from build123d import *

# Parameters (mm, degrees)
SKETCH1_R           = 14.2875
SKETCH1_R_2         = 2.4892
BOSS_EXTRUDE1_DEPTH = 2.54
FILLET1_R           = 7.62


with BuildPart() as part:
    # Sketch1 → Boss-Extrude1 (new body)
    with BuildSketch(Plane.XY):
        with BuildLine():
            Line((-76.2, -15.1892), (-76.2, -25.4))
            Line((-76.2, -25.4), (76.2, -25.4))
            Line((76.2, -25.4), (76.2, -15.1892))
            ThreePointArc((76.2, -15.1892), (73.7108, -12.7), (76.2, -10.2108))
            Line((76.2, -10.2108), (76.2, 133.35))
            Line((76.2, 133.35), (-76.2, 133.35))
            Line((-76.2, 133.35), (-76.2, -10.2108))
            ThreePointArc((-76.2, -10.2108), (-73.7108, -12.7), (-76.2, -15.1892))
        make_face()
        with Locations((0, 53.975)):
            Circle(SKETCH1_R, mode=Mode.SUBTRACT)
        with Locations((-63.5, -12.7)):
            Circle(SKETCH1_R_2, mode=Mode.SUBTRACT)
        with Locations((-50.8, -12.7)):
            Circle(SKETCH1_R_2, mode=Mode.SUBTRACT)
        with Locations((-38.1, -12.7)):
            Circle(SKETCH1_R_2, mode=Mode.SUBTRACT)
        with Locations((-25.4, -12.7)):
            Circle(SKETCH1_R_2, mode=Mode.SUBTRACT)
        with Locations((-12.7, -12.7)):
            Circle(SKETCH1_R_2, mode=Mode.SUBTRACT)
        with Locations((0, -12.7)):
            Circle(SKETCH1_R_2, mode=Mode.SUBTRACT)
        with Locations((12.7, -12.7)):
            Circle(SKETCH1_R_2, mode=Mode.SUBTRACT)
        with Locations((25.4, -12.7)):
            Circle(SKETCH1_R_2, mode=Mode.SUBTRACT)
        with Locations((38.1, -12.7)):
            Circle(SKETCH1_R_2, mode=Mode.SUBTRACT)
        with Locations((50.8, -12.7)):
            Circle(SKETCH1_R_2, mode=Mode.SUBTRACT)
        with Locations((63.5, -12.7)):
            Circle(SKETCH1_R_2, mode=Mode.SUBTRACT)
        with Locations((0, 109.855)):
            Circle(SKETCH1_R, mode=Mode.SUBTRACT)
    extrude(amount=BOSS_EXTRUDE1_DEPTH)

    # Fillet1
    fillet1_edges = [part.edges().sort_by_distance(p)[0] for p in [
        (76.2, -25.4, 1.27),
        (-76.2, -25.4, 1.27),
        (-76.2, 133.35, 1.27),
        (76.2, 133.35, 1.27),
    ]]
    fillet(fillet1_edges, radius=FILLET1_R)


solid = part.part
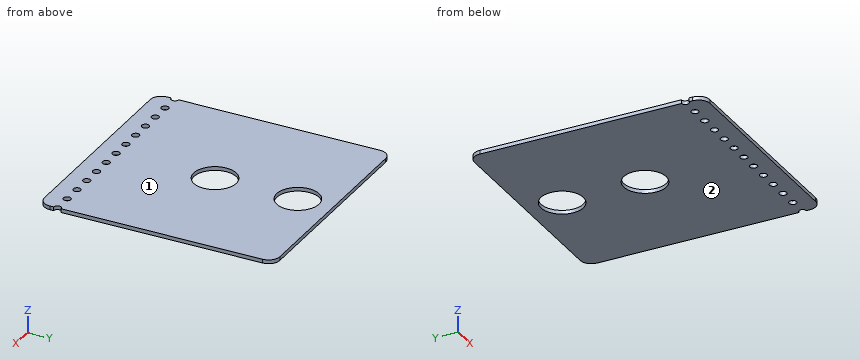
Design review of the part built by this model. Coordinates are the model's own, in mm. Face numbers are marked on the shaded views. Round coordinates to 2 decimals unless told otherwise and drop trailing zeros. Write each loop counter-clockwise with the first axis right and the second up, starting at its lowest first coordinate (ties: lowest second). Pieces come first, ordered by that corner, then holes. Notation, with made-up numbers: (-16.5, 23) - (-1.5, 23) arc R21 ccw to (-1.5, 58) - close; hole circle Ø10 at (71.5, 61.5). An arc over 180 degrees is marked (long way). Use a Markdown table: item, result. Add a question column.
1. We need section D-D (z = 1.1). Count the separate pieces of the cut face and the enclosed holes in it, then the cut area to 3 significant figures.
2. We need section A-A (x = -63.5). State the section outline as (y, z) points, then the cut area to 3 significant figures.
3. Wall thickness on probe 1 along Y at (x, z) = (0, 1.45); probe 2 along Y at (x, z) = (1, 1.4); probe 3 along Y at (x, z) = (-50.8, 1): over which ranges is each line inside the solid? List them lowest first.
4. We need section B-B (y = 46). State the section outline as (x, z) points.
5. Mouldability with a two-part tool opening along Z and no side actions: class the marked faces 1 and 2 as +Z half, -Z half, draft (parallel to the pull), parting line (faces both ways), or undercut.
6. We need section C-C (x = 0). State the section outline as (y, z) points, then the cut area to 3 significant figures.
Output:
| question | item | result |
|---|---|---|
| 1 | separate pieces | 1 |
| 1 | enclosed holes | 13 |
| 1 | area | 22,600 mm2 |
| 2 | outline | (-25.4, 0) - (-15.19, 0) - (-15.19, 2.54) - (-25.4, 2.54) - close; (-10.21, 0) - (133.35, 0) - (133.35, 2.54) - (-10.21, 2.54) - close |
| 2 | area | 391 mm2 |
| 3 | probe 1 | y = -25.4 to -15.19, -10.21 to 39.69, 68.26 to 95.57, 124.14 to 133.35 |
| 3 | probe 2 | y = -25.4 to -14.98, -10.42 to 39.72, 68.23 to 95.6, 124.11 to 133.35 |
| 3 | probe 3 | y = -25.4 to -15.19, -10.21 to 133.35 |
| 4 | outline | (-76.2, 0) - (-11.85, 0) - (-11.85, 2.54) - (-76.2, 2.54) - close; (11.85, 0) - (76.2, 0) - (76.2, 2.54) - (11.85, 2.54) - close |
| 5 | face 1 | +Z half |
| 5 | face 2 | -Z half |
| 6 | outline | (-25.4, 0) - (-15.19, 0) - (-15.19, 2.54) - (-25.4, 2.54) - close; (-10.21, 0) - (39.69, 0) - (39.69, 2.54) - (-10.21, 2.54) - close; (68.26, 0) - (95.57, 0) - (95.57, 2.54) - (68.26, 2.54) - close; (124.14, 0) - (133.35, 0) - (133.35, 2.54) - (124.14, 2.54) - close |
| 6 | area | 245 mm2 |
